Check sheet for the modelled part. Datum: model origin and axes. Units: mm. Coordinates: 2 decimals unless noted, no trailing zeros. Order: outer loops, then holes, each group sorted by start corner. A loop starts at its lowest first (then second) coordinate and runs counter-clockwise, first axis right, second up.
from build123d import *

# Parameters (mm, degrees)
F0_W     = 177.8
F0_H     = 63.5
F0_W_2   = 6.9088
F0_H_2   = 55.88
F1_DEPTH = 1.778
F2_W     = 20.7264
F2_H     = 55.88
F3_DEPTH = 1.778


with BuildPart() as f1:
    # F0 (on Front) → F1 (new body)
    with BuildSketch(Plane.XZ):
        Rectangle(F0_W, F0_H)
        Polygon((86.36, 27.94), (86.36, -27.94), (79.4512, -27.94), (72.5424, -27.94), (65.6336, -27.94), (58.7248, -27.94), (51.816, -27.94), (44.9072, -27.94), (37.9984, -27.94), (31.0896, -27.94), (24.1808, -27.94), (17.272, -27.94), (10.3632, -27.94), (3.4544, -27.94), (-3.4544, -27.94), (-10.3632, -27.94), (-17.272, -27.94), (-24.1808, -27.94), (-31.0896, -27.94), (-37.9984, -27.94), (-44.9072, -27.94), (-51.816, -27.94), (-58.7248, -27.94), (-65.6336, -27.94), (-72.5424, -27.94), (-79.4512, -27.94), (-86.36, -27.94), (-86.36, 27.94), (-79.4512, 27.94), (-72.5424, 27.94), (-65.6336, 27.94), (-58.7248, 27.94), (-51.816, 27.94), (-44.9072, 27.94), (-37.9984, 27.94), (-31.0896, 27.94), (-24.1808, 27.94), (-17.272, 27.94), (-10.3632, 27.94), (-3.4544, 27.94), (3.4544, 27.94), (10.3632, 27.94), (17.272, 27.94), (24.1808, 27.94), (31.0896, 27.94), (37.9984, 27.94), (44.9072, 27.94), (51.816, 27.94), (58.7248, 27.94), (65.6336, 27.94), (72.5424, 27.94), (79.4512, 27.94), align=None, mode=Mode.SUBTRACT)
        with Locations((-75.9968, 0)):
            Rectangle(F0_W_2, F0_H_2)
        with Locations((-62.1792, 0)):
            Rectangle(F0_W_2, F0_H_2)
        with Locations((-48.3616, 0)):
            Rectangle(F0_W_2, F0_H_2)
        with Locations((-34.544, 0)):
            Rectangle(F0_W_2, F0_H_2)
        with Locations((-20.7264, 0)):
            Rectangle(F0_W_2, F0_H_2)
        with Locations((-6.9088, 0)):
            Rectangle(F0_W_2, F0_H_2)
        with Locations((6.9088, 0)):
            Rectangle(F0_W_2, F0_H_2)
        with Locations((20.7264, 0)):
            Rectangle(F0_W_2, F0_H_2)
        with Locations((34.544, 0)):
            Rectangle(F0_W_2, F0_H_2)
        with Locations((48.3616, 0)):
            Rectangle(F0_W_2, F0_H_2)
        with Locations((62.1792, 0)):
            Rectangle(F0_W_2, F0_H_2)
        with Locations((75.9968, 0)):
            Rectangle(F0_W_2, F0_H_2)
    extrude(amount=F1_DEPTH)

    # F2 (on face) → F3 (join)
    with BuildSketch(Plane.XZ.offset(1.778)):
        with Locations((-75.9968, 0)):
            Rectangle(F2_W, F2_H)
    extrude(amount=-F3_DEPTH)


solid = f1.part
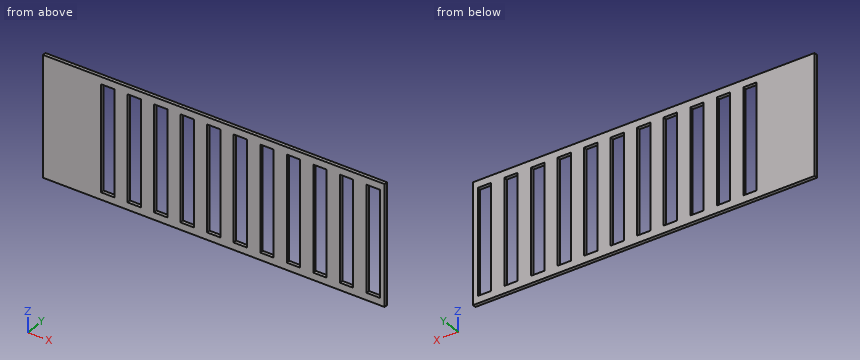
(1) Cross-section at B-B (z = -1.5). Count the separate pieces of the cut face and the enclosed holes in it, and give its area (3 significant figures).
Filled in:
separate pieces: 12
enclosed holes: 0
area: 181 mm2
(2) Thickness scan on probe 1 along Z at (x, y) = (-29, -1.7). Record the ranges inside material, lowest first.
Filled in:
probe 1: z = -31.75 to -27.94, 27.94 to 31.75
(3) Go/stop test with a flat-tipped pin: P1, Ø5, axis at x = -69, z = 5, coming from the +Y side. Record where the tip stops, or that it passes through.
Filled in:
P1: stops at y = 0
(4) Cross-section at A-A (x = -41.5). Enter the section's corners in (y, z), and give its area (3 significant figures).
Filled in:
outline: (-1.78, -31.75) - (0, -31.75) - (0, -27.94) - (-1.78, -27.94) - close; (-1.78, 27.94) - (0, 27.94) - (0, 31.75) - (-1.78, 31.75) - close
area: 13.5 mm2
